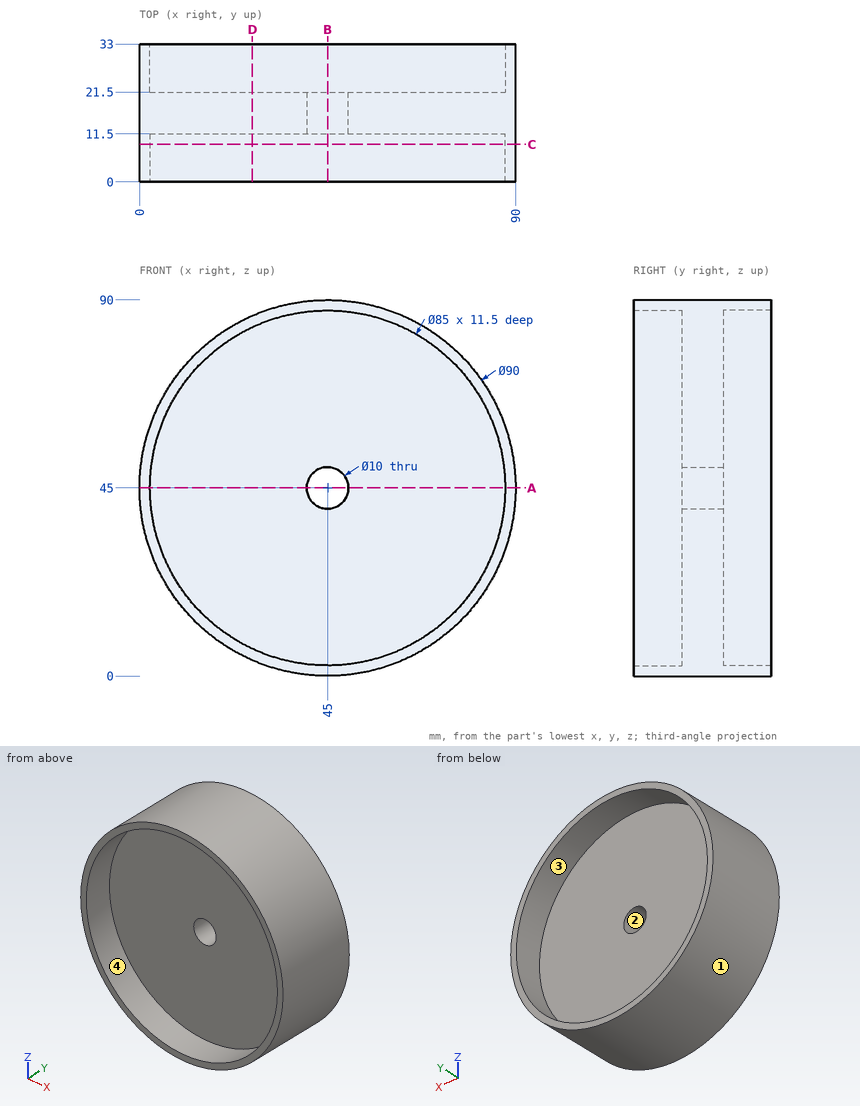
The drawing under review shows one solid part. Ordinate dimensions are in mm from its lowest x, y, z. A direction names the side the tool comes from. Coordinates: 2 decimals unless noted, no trailing zeros. Write each loop counter-clockwise with the first axis right and the second up, starting at its lowest first coordinate (ties: lowest second). Pieces come first, ordered by that corner, then holes. Notation, with made-up numbers: M 41.25,-36.75 L 94.25,-36.75 A16 ccw 94.25,-5.75 Z; hole C 4,10.25 d2. An arc over 180 degrees is marked long. Answer as a JSON object with one key per item and string values.
Item 1: Draft analysis for pull direction Z (two halves, no side actions). For the marked faces 1 and 2, state which applies: pulls with the +Z half, pulls with the -Z half, needs draft (parallel to the pull), parting line crosses it, or undercut.
Outcome:
{"face 1": "parting line crosses it", "face 2": "undercut"}
Item 2: Wall thickness on probe 1 along Z at (x, y) = (45, 7.5); probe 2 along Y at (x, z) = (77.5, 48); probe 3 along Z at (x, y) = (73, 29): over which ranges is each line inside the solid? List them lowest first.
Outcome:
{"probe 1": "0 to 2.5, 87.5 to 90", "probe 2": "11.5 to 21.5", "probe 3": "9.77 to 13.03, 76.97 to 80.23"}
Item 3: Insertion check: pin 1 Ø4 at (x, z) = (19.5, 67) entering from -Y; pin 2 Ø4 at (x, y) = (50.5, 13.5) entering from -Z; pin 3 Ø6 at (x, z) = (45, 45) entering from +Y; pin 4 Ø4 at (x, y) = (75, 25) entering from +Z. Each pin has a flat end and moves straight along its axis. Give the tip position at first contact, or say it passes through.
Outcome:
{"pin 1": "y = 11.5", "pin 2": "z = 0.14", "pin 3": "through", "pin 4": "z = 80.23"}
Item 4: Machinability: for the marked faces 3 and 4, which of the approach directions +Z, -Z, +X, -X, +Y, -Y give a long, thin tool a straight path to every point of the face, cutting with its end or side? Answer none if there is none.
Outcome:
{"face 3": "+Y", "face 4": "-Y"}
Item 5: Add section A-A, the plane z = 45. Give the boundary of the cut face in (x, y).
Outcome:
{"outline": "M 0,0 L 2.5,0 L 2.5,11.5 L 40,11.5 L 40,21.5 L 2.5,21.5 L 2.5,33 L 0,33 Z; M 50,11.5 L 87.5,11.5 L 87.5,0 L 90,0 L 90,33 L 87.5,33 L 87.5,21.5 L 50,21.5 Z"}
Item 6: Add section C-C, the plane y = 9. Give the boundary of the cut face in (x, z), and give its area (3 significant figures).
Outcome:
{"outline": "C 45,45 d90; hole C 45,45 d85", "area": "687 mm²"}
Item 7: Add section D-D, the plane x = 27. Give the boundary of the cut face in (y, z), and give its area (3 significant figures).
Outcome:
{"outline": "M 0,3.76 L 33,3.76 L 33,6.5 L 21.5,6.5 L 21.5,83.5 L 33,83.5 L 33,86.24 L 0,86.24 L 0,83.5 L 11.5,83.5 L 11.5,6.5 L 0,6.5 Z", "area": "951 mm²"}
Item 8: Add section B-B, the plane x = 45. Give the boundary of the cut face in (y, z), and give its area (3 significant figures).
Outcome:
{"outline": "M 0,0 L 33,0 L 33,2.5 L 21.5,2.5 L 21.5,40 L 11.5,40 L 11.5,2.5 L 0,2.5 Z; M 0,87.5 L 11.5,87.5 L 11.5,50 L 21.5,50 L 21.5,87.5 L 33,87.5 L 33,90 L 0,90 Z", "area": "915 mm²"}
